Could you check a few things on this drawing? It's one solid part, dimensions in mm from its lowest x, y, z. A direction names the side the tool comes from. Coordinates: 2 decimals unless noted, no trailing zeros. Loops run counter-clockwise (first coordinate to the right, second up) from the corner with the lowest first, then second, coordinate; pieces in that order, holes last. Notation, with made-up numbers: (86, -37) -> (93, -37) arc R19 cw to (93, -5) -> close; hole circle Ø3 at (6.25, 32.25). An arc over 180 degrees is marked (long way). One line per question, with ' | ' between items. Start each with the question number.
(1) If we mould it in two halves opening along X, with no side actions, what happens to the marked faces 1, 2 and 3? For each: pulls with the +X half, pulls with the -X half, needs draft (parallel to the pull), parting line crosses it, or undercut.
(2) Which directions (+Z, -Z, +X, -X, +Y, -Y) give clear straight access to the entire face, cutting with the end or side of a thin tool? Please do the marked faces 4 and 5.
(3) I'm going to push flat-ended pins straight in: pin 1 Ø1.5 at (x, z) = (8, 3.5) entering from +Y; pin 2 Ø2 at (y, z) = (9, 4) entering from +X; pin 3 Ø1 at (y, z) = (7, 6) entering from -X. Where does each tip first touch, or does it pass through?
(4) Suppose I cut it at C-C (y = 5). Please give me the cut outline in (x, z), plus the area to 3 significant figures.
(5) Suppose I cut it at A-A (x = 5). Please give me the cut outline in (y, z), plus the area to 3 significant figures.
(6) If I drill on line 1 along Y through (x, z) = (3, 4.5); line 2 along X through (y, z) = (5.5, 6); line 3 along X through (y, z) = (9, 6.75), over which ranges is the centre line in solid material (lowest first)?
(7) Suppose I cut it at D-D (z = 6.25). Please give me the cut outline in (x, y).
(8) Suppose I cut it at B-B (z = 5). Please give me the cut outline in (x, y), plus the area to 3 significant figures.
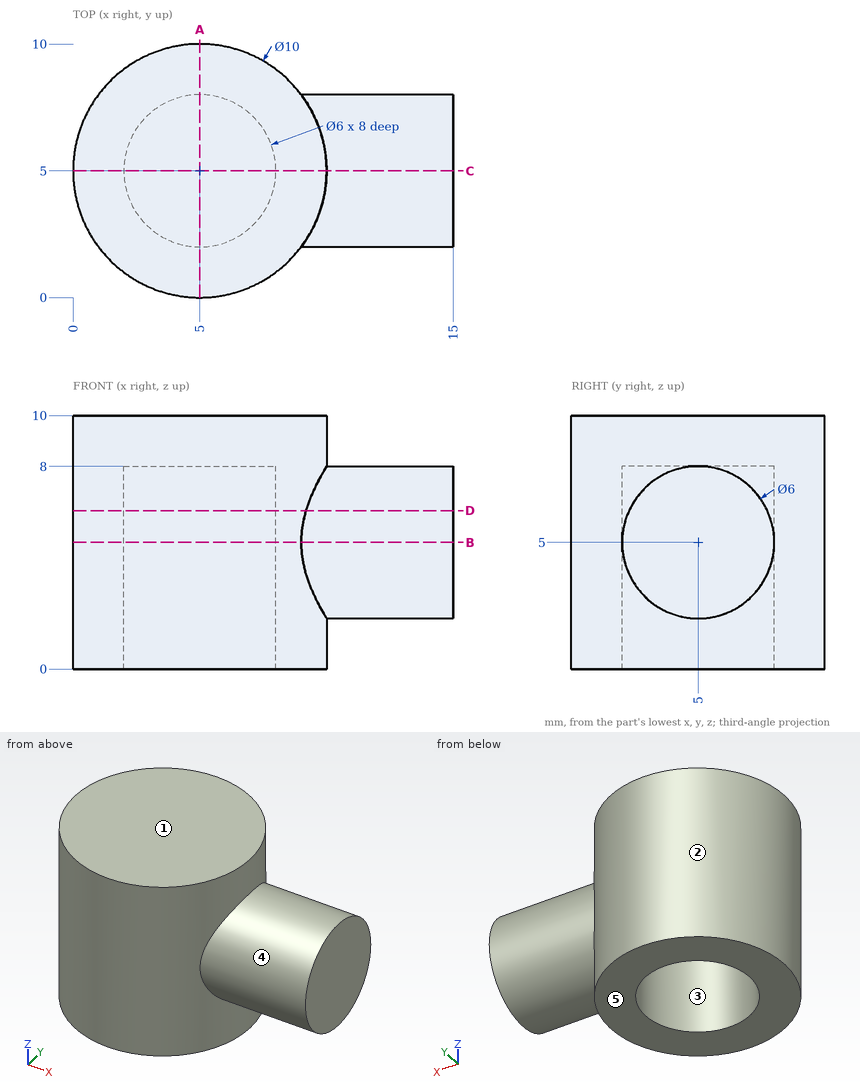
Checks:
1) face 1: needs draft | face 2: parting line crosses it | face 3: undercut
2) face 4: +X | face 5: -Z, +X, -X, +Y, -Y
3) pin 1: stops at y = 9.47 | pin 2: stops at x = 9 | pin 3: stops at x = 0.23
4) outline: (0, 0) -> (2, 0) -> (2, 8) -> (8, 8) -> (8, 0) -> (10, 0) -> (10, 2) -> (15, 2) -> (15, 8) -> (10, 8) -> (10, 10) -> (0, 10) -> close | area: 82.0 mm^2
5) outline: (0, 0) -> (2, 0) -> (2, 8) -> (8, 8) -> (8, 0) -> (10, 0) -> (10, 10) -> (0, 10) -> close | area: 52.0 mm^2
6) line 1: y = 0.42 to 2.76, 7.24 to 9.58 | line 2: x = 0.03 to 2.04, 7.96 to 15 | line 3: x = 2 to 8
7) outline: (9.19, 2.27) -> (15, 2.27) -> (15, 7.73) -> (9.19, 7.73) arc R5 ccw (long way) to start; hole circle Ø6 at (5, 5)
8) outline: (9, 2) -> (15, 2) -> (15, 8) -> (9, 8) arc R5 ccw (long way) to start; hole circle Ø6 at (5, 5) | area: 82.2 mm^2
